For this review, take the finished solid that the model builds, in its own axes (mm). Give positions to 0.01 mm unless a question says otherwise; leave off trailing zeros. Order: outer loops, then holes, each group sorted by start corner. A loop starts at its lowest first (then second) coordinate and runs counter-clockwise, first axis right, second up. Notation, with made-up numbers: (77, 50) -> (88, 50) arc R19 cw to (88, 79) -> close; hole circle Ø5 at (-32, 79.5). An arc over 180 degrees is marked (long way). Return JSON: item names as keys, results as strings. Group by question number.
1) Insertion check: P1, Ø1.5, axis at y = -5, z = 1, coming from the +X side; P2, Ø1.5, axis at x = 37.5, z = 1.5, coming from the -Y side; P3, Ø2, axis at x = -37, z = 1.5, coming from the -Y side. Each pin has a flat end and moves straight along its axis. Give the tip position at first contact, or say it passes through.
2) To check wall thickness, follow line 1 along X through (y, z) = (-30, 2); line 2 along X through (y, z) = (-28, 1.25); line 3 along Y through (x, z) = (8, 3.85). State the ranges of each line that lie inside material, in increasing order.
3) Add section A-A (z = 1.05). Give the boundary of the cut face in (x, y), then the cut area to 3 significant figures.
from build123d import *

# Parameters (mm, degrees)
BOSS_EXTRUDE1_DEPTH = 4
CHAMFER1_SIZE       = 1.5


with BuildPart() as part:
    # Sketch1 → Boss-Extrude1 (new body)
    with BuildSketch(Plane.XY):
        with BuildLine():
            Line((-54.748665604, 40.101038648), (59.035797152, 20.037767879))
            ThreePointArc((59.035797152, 20.037767879), (76.21528885, 10.119183723), (83, -8.521656958))
            Line((83, -8.521656958), (83, -38.521656958))
            ThreePointArc((83, -38.521656958), (76.697736677, -50.742515222), (63.086749774, -52.694164578))
            ThreePointArc((63.086749774, -52.694164578), (2.15504295, -40.457474253), (-59.828407224, -44.980901185))
            ThreePointArc((-59.828407224, -44.980901185), (-80.743414188, -39.941876053), (-90, -20.521656958))
            Line((-90, -20.521656958), (-90, 10.521656958))
            ThreePointArc((-90, 10.521656958), (-79.270878905, 33.530331398), (-54.748665604, 40.101038648))
        make_face()
    extrude(amount=BOSS_EXTRUDE1_DEPTH)

    # Chamfer1
    chamfer1_edges = [part.edges().sort_by_distance(p)[0] for p in [
        (-80.743414188, -39.941876053, 4),
        (2.15504295, -40.457474253, 4),
        (76.697736677, -50.742515222, 4),
        (83, -23.521656958, 4),
        (76.21528885, 10.119183723, 4),
        (2.143565774, 30.069403264, 4),
        (-79.270878905, 33.530331398, 4),
        (-90, -5, 4),
    ]]
    chamfer(chamfer1_edges, length=CHAMFER1_SIZE)


solid = part.part
Evaluation:
{
 "1": {"P1": "x = 82.87", "P2": "y = -45.62", "P3": "y = -41.45"},
 "2": {"line 1": "-88.13 to 83", "line 2": "-88.86 to 83", "line 3": "-39.54 to 27.67"},
 "3": {"outline": "(-90, -20.52) arc R25 ccw to (-59.83, -44.98) arc R230 cw to (63.09, -52.69) arc R15 ccw to (83, -38.52) -> (83, -8.52) arc R29 ccw to (59.04, 20.04) -> (-54.75, 40.1) arc R30.04 ccw to (-90, 10.52) -> close", "area": "12,500 mm^2"}
}
